Input: dimensioned drawing with shaded views. Units: mm. Origin: part minimum x, y, z. A direction names the side the tool comes from. Coordinates: 2 decimals unless noted, no trailing zeros. Order: outer loops, then holes, each group sorted by start corner. A loop starts at its lowest first (then second) coordinate and runs counter-clockwise, first axis right, second up. Notation, with made-up numbers: M 12.25,79.5 L 46.25,79.5 A32 ccw 46.25,115.5 Z; hole C 88,78.25 d10. An arc over 180 degrees is marked long. Write item = value, one per line.
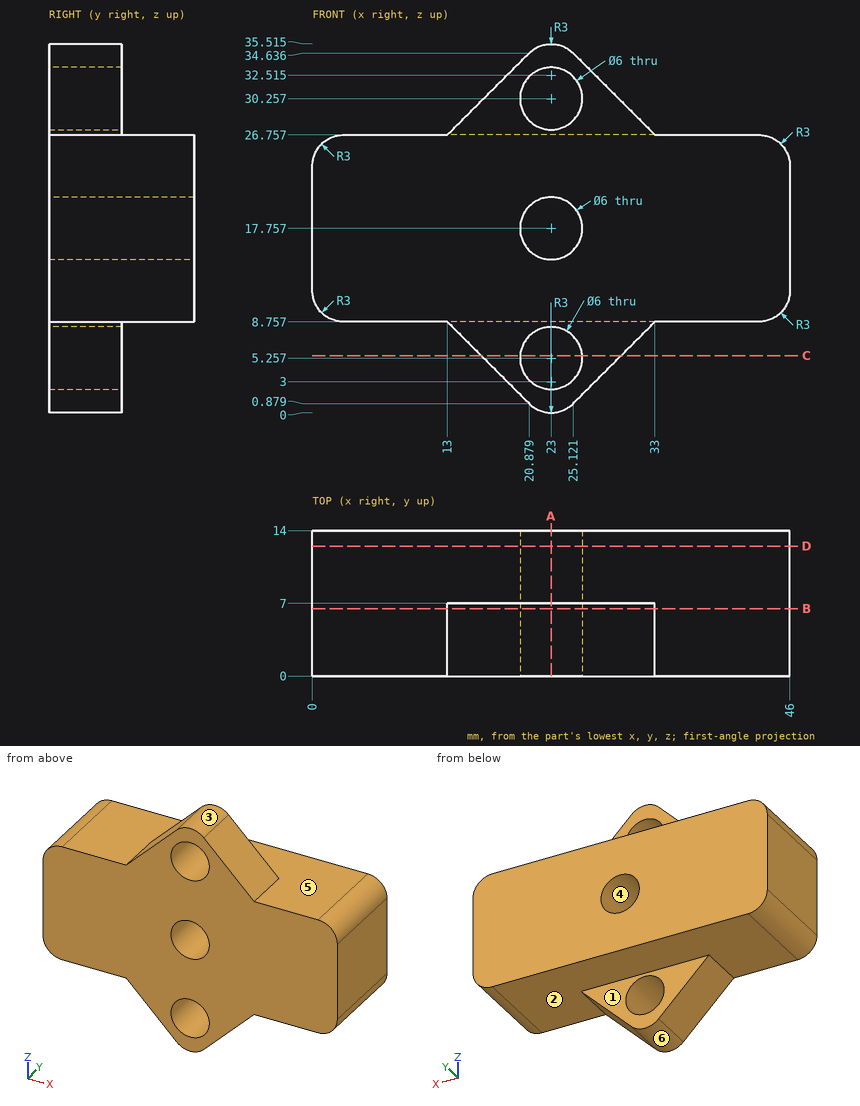
1) Pin query (flat end, axial travel): pin 1 (9.5 mm diameter, centred on x = 23, z = 5.26, fed in from -Y); pin 2 (4 mm diameter, centred on x = 38.5, y = 12.5, fed in from +Z); pin 3 (2.5 mm diameter, centred on x = 23.5, z = 31, fed in from +Y); pin 4 (1 mm diameter, centred on x = 31, y = 2, fed in from -Z). Return the tip coordinate at first contact, or that it passes through.
Numbers:
pin_1 = 0
pin_2 = 26.76
pin_3 = through
pin_4 = 6.26
2) Line query: L1, parallel to X at y = 8.75, z = 18; L2, parallel to Y at x = 27.5, z = 28.5; L3, parallel to Z at x = 20.5, y = 7.5 (1 decimal). Output: solid intervals per line, ascending.
Numbers:
L1 = 0 to 20.01, 25.99 to 46
L2 = 0 to 7
L3 = 8.8 to 16.1, 19.4 to 26.8
3) Section C-C, the plane z = 5.5. Return loops of the section in (x, y).
Numbers:
outline = M 16.26,0 L 20.01,0 L 20.01,7 L 16.26,7 Z; M 25.99,0 L 29.74,0 L 29.74,7 L 25.99,7 Z
4) Section B-B, the plane y = 6.5. Return loops of the section in (x, z) (1 decimal).
Numbers:
outline = M 0,11.8 A3 ccw 3,8.8 L 13,8.8 L 20.9,0.9 A3 ccw 25.1,0.9 L 33,8.8 L 43,8.8 A3 ccw 46,11.8 L 46,23.8 A3 ccw 43,26.8 L 33,26.8 L 25.1,34.6 A3 ccw 20.9,34.6 L 13,26.8 L 3,26.8 A3 ccw 0,23.8 Z; hole C 23,5.3 d6; hole C 23,17.8 d6; hole C 23,30.3 d6
5) Section A-A, the plane x = 23. Return loops of the section in (y, z) (1 decimal), and give its area (3 significant figures).
Numbers:
outline = M 0,0 L 7,0 L 7,2.3 L 0,2.3 Z; M 0,8.3 L 7,8.3 L 7,8.8 L 14,8.8 L 14,14.8 L 0,14.8 Z; M 0,20.8 L 14,20.8 L 14,26.8 L 7,26.8 L 7,27.3 L 0,27.3 Z; M 0,33.3 L 7,33.3 L 7,35.5 L 0,35.5 Z
area = 207 mm²
6) Set-up query: the marked faces 5 and 6. Return all of +Z, -Z, +X, -X, +Y, -Y with unobstructed straight access to the full face (end or side cutting, diameter ignored); none if empty.
Numbers:
face_5 = +Z, +Y
face_6 = -Z, +Y, -Y
7) Section D-D, the plane y = 12.5. Return loops of the section in (x, z).
Numbers:
outline = M 0,11.76 A3 ccw 3,8.76 L 43,8.76 A3 ccw 46,11.76 L 46,23.76 A3 ccw 43,26.76 L 3,26.76 A3 ccw 0,23.76 Z; hole C 23,17.76 d6
8) Mould query, pull axis Z, two halves, no side actions, for the marked faces 1, 2, 3 and 4. Classes: pulls with the +Z half, pulls with the -Z half, needs draft (parallel to the pull), parting line crosses it, or undercut.
Numbers:
face_1 = needs draft
face_2 = pulls with the -Z half
face_3 = pulls with the +Z half
face_4 = undercut
